from build123d import *

# Parameters (mm, degrees)
SKETCH_4_R               = 10
EXTRUDE_2_DEPTH          = 2.5
SKETCH_7_R               = 4.4
EXTRUDE_3_DEPTH          = 2
SKETCH_8_R               = 3
CUT_EXTRUDE_10_DEPTH     = 3
EXTRUDE_5_DEPTH          = 2
PATTERN_CIRCULAR_1_COUNT = 24
HOLE_WIZARD_M3_1_D       = 2.5
CUT_EXTRUDE_11_REACH     = 16.841
SKETCH_18_R              = 1.5


with BuildPart() as part:
    # Sketch 4 → Extrude 2 (new body)
    with BuildSketch(Plane(origin=(0, 0, 0), x_dir=(1, 0, 0), z_dir=(0, 1, 0))):
        with Locations(Location((0, 0, 0), (0, 0, 270))):
            Circle(SKETCH_4_R)
    extrude(amount=EXTRUDE_2_DEPTH)

    # Sketch 7 → Extrude 3 (add)
    with BuildSketch(Plane(origin=(0, 2.5, 0), x_dir=(1, 0, 0), z_dir=(0, 1, 0))):
        with Locations(Location((0, 0, 0), (0, 0, 270))):
            Circle(SKETCH_7_R)
    extrude(amount=EXTRUDE_3_DEPTH)

    # Sketch 8 → Cut-Extrude 10 (cut)
    with BuildSketch(Plane(origin=(0, 4.5, 0), x_dir=(1, 0, 0), z_dir=(0, 1, 0))):
        with Locations(Location((0, 0, 0), (0, 0, 270))):
            Circle(SKETCH_8_R)
    extrude(amount=-CUT_EXTRUDE_10_DEPTH, mode=Mode.SUBTRACT)

    # Sketch 14 → Extrude 5 (add)
    with BuildSketch(Plane(origin=(0, 4.5, 0), x_dir=(1, 0, 0), z_dir=(0, 1, 0))):
        with BuildLine():
            Line((2.976910005, -0.371492698), (2.495792863, -0.23538136))
            Line((2.495792863, -0.23538136), (2.495792863, 0.032272898))
            Line((2.495792863, 0.032272898), (2.995792863, 0.158824181))
            ThreePointArc((2.995792863, 0.158824181), (2.998100046, -0.106752588), (2.976910005, -0.371492698))
        make_face()
    extrude_5 = extrude(amount=-EXTRUDE_5_DEPTH)

    # Pattern Circular 1: Extrude 5 ×24 about axis
    pattern_circular_1_axis = Axis((0, 0, 0), (0, 1, 0))
    for i in range(1, PATTERN_CIRCULAR_1_COUNT):
        add(extrude_5.rotate(pattern_circular_1_axis, i * 360 / PATTERN_CIRCULAR_1_COUNT))

    # Hole Wizard M3 _1 (through all)
    with Locations(Plane(origin=(0, 0, 0), x_dir=(-1, 0, 0), z_dir=(0, -1, 0))):
        with Locations((0, -7), (7, 0), (0, 7), (-7, 0)):
            Hole(HOLE_WIZARD_M3_1_D / 2)

    # Sketch 18 → Cut-Extrude 11 (cut, up to next)
    with BuildSketch(Plane.XZ, mode=Mode.PRIVATE) as cut_extrude_11_sk1:
        with Locations(Location((0, 0, 0), (0, 0, 270))):
            Circle(SKETCH_18_R)
    cut_extrude_11_tool1 = extrude(cut_extrude_11_sk1.sketch, amount=-CUT_EXTRUDE_11_REACH, mode=Mode.PRIVATE) & part.part
    add(cut_extrude_11_tool1.solids().sort_by_distance((0, 0, 0))[0], mode=Mode.SUBTRACT)


solid = part.part
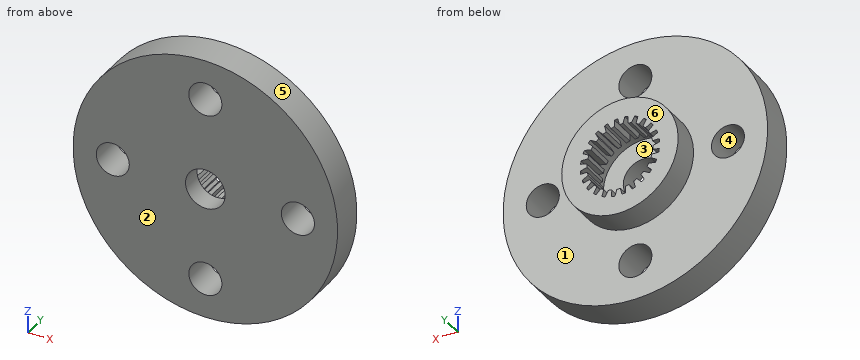
Here's how the part is built. I have some questions about the finished solid (model axes, mm). Face numbers are marked on the shaded views. A direction names the side the tool comes from. Give positions to 0.01 mm unless a question says otherwise; leave off trailing zeros. Loops run counter-clockwise (first coordinate to the right, second up) from the corner with the lowest first, then second, coordinate; pieces in that order, holes last. Notation, with made-up numbers: (5, -8) -> (31, -8) arc R27 cw to (31, 31) -> close; hole circle Ø4 at (64, 52). An arc over 180 degrees is marked (long way). One line per item, written item: value.
Q1. Suppose I cut it at C-C on y = 0.65. Please give me the cut outline in (x, z), then the cut area to 3 significant figures.
Answers follow:
outline: circle Ø20 at (0, 0); hole circle Ø2.5 at (-7, 0); hole circle Ø3 at (0, 0); hole circle Ø2.5 at (0, -7); hole circle Ø2.5 at (0, 7); hole circle Ø2.5 at (7, 0)
area: 287 mm^2
Q2. If I drill on line 1 along Y through (x, z) = (-2, 2); line 2 along X through (y, z) = (1.65, 0.5); line 3 along Y through (x, z) = (8.5, 5), over which ranges is the centre line in solid material (lowest first)?
Answers follow:
line 1: 0 to 1.5, 2.5 to 4.5
line 2: -9.99 to -8.15, -5.85 to -2.96, 2.96 to 5.85, 8.15 to 9.99
line 3: 0 to 2.5
Q3. I'm going to push flat-ended pins straight in: pin 1 Ø1 at (x, z) = (5.5, -1) entering from +Y; pin 2 Ø8 at (x, z) = (-3.5, -4) entering from -Y; pin 3 Ø1.5 at (x, y) = (3.5, 3) entering from +Z. Where does each tip first touch, or does it pass through?
Answers follow:
pin 1: y = 2.5
pin 2: y = 0
pin 3: z = 9.56
Q4. We'd pull the mould along X, two halves only. Please class the marked faces 4, 5 and 6: pulls with the +X half, pulls with the -X half, needs draft (parallel to the pull), parting line crosses it, or undercut.
Answers follow:
face 4: undercut
face 5: parting line crosses it
face 6: needs draft
Q5. On a 3-axis mill with a long thin cutter (end or side, diameter ignored), from which of +Z, -Z, +X, -X, +Y, -Y can I reach the whole of each face in a straight line? I mean the marked faces 1, 2 and 3. Say none if no direction works.
Answers follow:
face 1: +Y
face 2: +Z, -Z, +X, -X, -Y
face 3: none
Q6. Suppose I cut it at B-B on x = 7. Please give me the cut outline in (y, z).
Answers follow:
outline: (0, -7.14) -> (2.5, -7.14) -> (2.5, -1.25) -> (0, -1.25) -> close; (0, 1.25) -> (2.5, 1.25) -> (2.5, 7.14) -> (0, 7.14) -> close
Q7. Suppose I cut it at D-D on y = 2.2. Please give me the cut outline in (x, z).
Answers follow:
outline: circle Ø20 at (0, 0); hole circle Ø2.5 at (-7, 0); hole circle Ø6 at (0, 0); hole circle Ø2.5 at (0, -7); hole circle Ø2.5 at (0, 7); hole circle Ø2.5 at (7, 0)
Q8. Suppose I cut it at A-A on z = -8. Please give me the cut outline in (x, y), then the cut area to 4 significant figures.
Answers follow:
outline: (-6, 0) -> (-0.75, 0) -> (-0.75, 2.5) -> (-6, 2.5) -> close; (0.75, 0) -> (6, 0) -> (6, 2.5) -> (0.75, 2.5) -> close
area: 26.25 mm^2
